For this review, use the dimensioned drawing (mm, ordinates from the lowest corner) and the shaded views. Coordinates: 2 decimals unless noted, no trailing zeros. Write each loop counter-clockwise with the first axis right and the second up, starting at its lowest first coordinate (ties: lowest second). Pieces come first, ordered by that corner, then holes. Notation, with made-up numbers: M 86,11.5 L 128,11.5 A15 ccw 128,36.5 Z; hole C 33,48 d9. An arc over 180 degrees is marked long. Return JSON: item names as keys, results as strings.
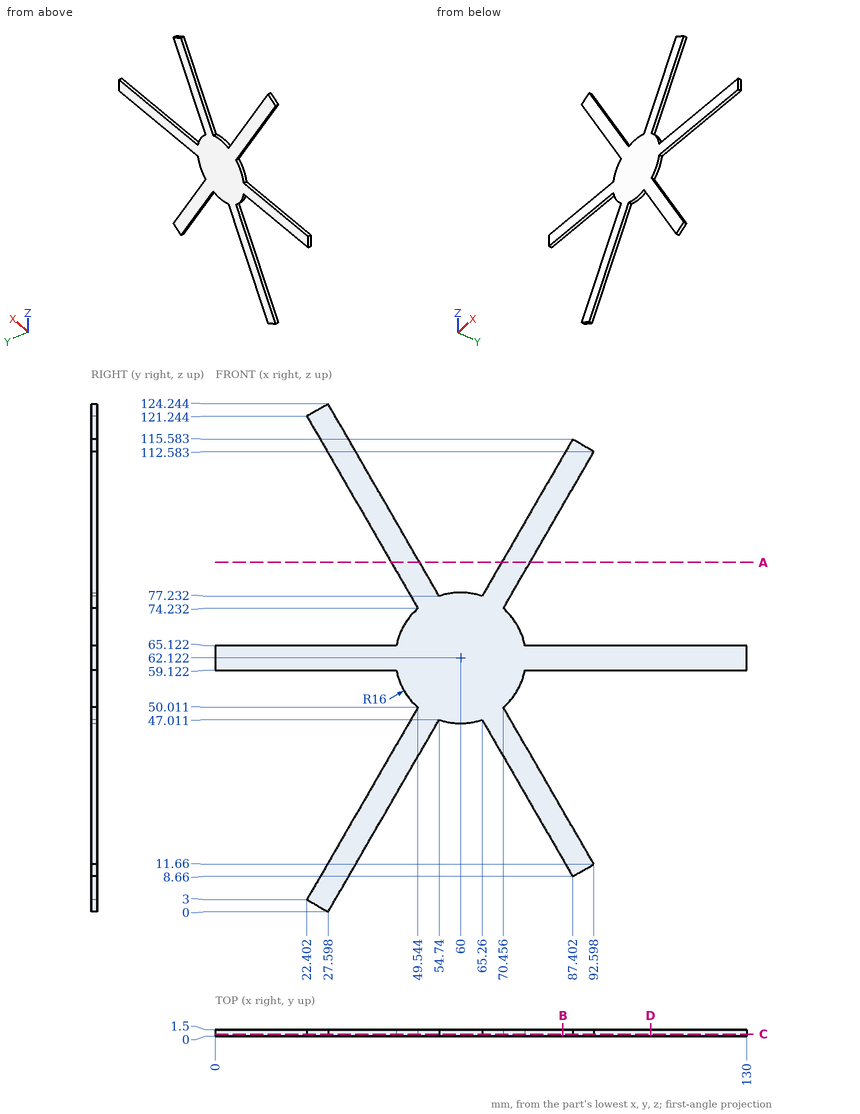
1. Clearance check with a flat-ended pin moving along its axis: pin 1 Ø0.8 at (x, y) = (90.5, 0.5) entering from -Z. State where the tip first meets the part, or that it passes through.
Checks:
{"pin 1": "z = 10.22"}
2. We need section C-C (y = 0.45). State the section outline as (x, z) points.
Checks:
{"outline": "M 0,59.12 L 44.28,59.12 A16 ccw 49.54,50.01 L 22.4,3 L 27.6,0 L 54.74,47.01 A16 ccw 65.26,47.01 L 87.4,8.66 L 92.6,11.66 L 70.46,50.01 A16 ccw 75.72,59.12 L 130,59.12 L 130,65.12 L 75.72,65.12 A16 ccw 70.46,74.23 L 92.6,112.58 L 87.4,115.58 L 65.26,77.23 A16 ccw 54.74,77.23 L 27.6,124.24 L 22.4,121.24 L 49.54,74.23 A16 ccw 44.28,65.12 L 0,65.12 Z"}
3. We need section B-B (x = 85). State the section outline as (y, z) points.
Checks:
{"outline": "M 0,12.82 L 1.5,12.82 L 1.5,24.82 L 0,24.82 Z; M 0,59.12 L 1.5,59.12 L 1.5,65.12 L 0,65.12 Z; M 0,99.42 L 1.5,99.42 L 1.5,111.42 L 0,111.42 Z"}
4. We need section A-A (z = 85.5). State the section outline as (x, y) points.
Checks:
{"outline": "M 43.04,0 L 49.97,0 L 49.97,1.5 L 43.04,1.5 Z; M 70.03,0 L 76.96,0 L 76.96,1.5 L 70.03,1.5 Z"}
5. We need section D-D (x = 106.5). State the section outline as (y, z) points.
Checks:
{"outline": "M 0,59.12 L 1.5,59.12 L 1.5,65.12 L 0,65.12 Z"}
6. Wall thickness on L1, parallel to Z at x = 26.5, y = 1.4 (1 decimal); L2, parallel to Z at x = 119, y = 0.75; L3, parallel to X at y = 0.9, z = 23: over which ranges is each line inside the solid? List them lowest first. Write a range as from..to.
Checks:
{"L1": "0.6..10.1, 59.1..65.1, 114.1..123.6", "L2": "59.12..65.12", "L3": "33.95..40.88, 79.12..86.05"}
